CAD build for the part. Positions are in the model's coordinates, mm. Give positions to 0.01 mm unless a question says otherwise; leave off trailing zeros. Loops run counter-clockwise (first coordinate to the right, second up) from the corner with the lowest first, then second, coordinate; pieces in that order, holes last. Notation, with made-up numbers: M -21.75,38 L 3.25,38 A16 cw 3.25,54 Z; hole C 59.5,36.5 d7. An arc over 180 degrees is marked long. Answer as CSV lines item,"result".
```python
from build123d import *

# Parameters (mm, degrees)
F0_R     = 1.7
F1_DEPTH = 5


with BuildPart() as f1:
    # F0 (on Top) → F1 (new body)
    with BuildSketch(Plane.XY):
        with Locations((-11.34986, 17.466265)):
            Circle(F0_R)
        Polygon((-2.84986, 22.466265), (-21.74986, 22.466265), (-21.74986, 12.466265), (-2.84986, 12.466265), (-2.84986, 17.466265), align=None)
        with Locations((-11.34986, 17.466265)):
            Circle(F0_R, mode=Mode.SUBTRACT)
        with BuildLine():
            ThreePointArc((7.35014, 17.466265), (5.65014, 19.166265), (3.95014, 17.466265))
            ThreePointArc((3.95014, 17.466265), (5.65014, 15.766265), (7.35014, 17.466265))
        make_face()
        Polygon((16.05014, 22.466265), (-2.84986, 22.466265), (-2.84986, 17.466265), (-2.84986, 12.466265), (16.05014, 12.466265), align=None)
        with BuildLine():
            ThreePointArc((7.35014, 17.466265), (5.65014, 15.766265), (3.95014, 17.466265))
            ThreePointArc((3.95014, 17.466265), (5.65014, 19.166265), (7.35014, 17.466265))
        make_face(mode=Mode.SUBTRACT)
    extrude(amount=F1_DEPTH)


solid = f1.part
```
Q1. Cut at B-B (x = -11). Write the cut outline in (y, z).
Solution:
outline,"M 12.47,0 L 15.8,0 L 15.8,5 L 12.47,5 Z; M 19.13,0 L 22.47,0 L 22.47,5 L 19.13,5 Z"
Q2. Wall check: line 1 (X direction, y = 18.25, z = 2.85); line 2 (X direction, y = 17, z = 4.3); line 3 (Y direction, x = -10, z = 3.75). Give the ranges that are in metal, low to high. Write a range as [from, to].
Solution:
line 1,"x = [-21.75, -12.86], [-9.84, 4.14], [7.16, 16.05]"
line 2,"x = [-21.75, -12.98], [-9.72, 4.02], [7.28, 16.05]"
line 3,"y = [12.47, 16.43], [18.5, 22.47]"
Q3. Mould opens along Y. For faces 1 (the flat face through (-3, 12.466, 2)), 2 (the cylindrical face through (-10.44, 18.9, 2.46)), 3 (the flat face through (-3, 18, 5)) say: released by +Y, released by -Y, zero draft, split by the parting line, or undercut.
Solution:
face 1,"released by -Y"
face 2,"undercut"
face 3,"zero draft"
Q4. Pin check, flat tips, straight feed: P1, Ø2, axis at x = -11.35, y = 17.47, coming from the +Z side; P2, Ø5.5, axis at x = 5.65, y = 17.47, coming from the +Z side. Stop position of each tip, or through.
Solution:
P1,"passes through"
P2,"stops at z = 5"
Q5. Cut at C-C (z = 4.1). Write the cut outline in (x, y), and give its area (3 significant figures).
Solution:
outline,"M -21.75,12.47 L 16.05,12.47 L 16.05,22.47 L -21.75,22.47 Z; hole C -11.35,17.47 d3.4; hole C 5.65,17.47 d3.4"
area,"360 mm²"
Q6. Cut at A-A (y = 18.75). Write the cut outline in (x, z), and give its area (3 significant figures).
Solution:
outline,"M -21.75,0 L -12.46,0 L -12.46,5 L -21.75,5 Z; M -10.24,0 L 4.54,0 L 4.54,5 L -10.24,5 Z; M 6.76,0 L 16.05,0 L 16.05,5 L 6.76,5 Z"
area,"167 mm²"
Q7. Cut at D-D (y = 16.75). Write the cut outline in (x, z).
Solution:
outline,"M -21.75,0 L -12.89,0 L -12.89,5 L -21.75,5 Z; M -9.81,0 L 4.11,0 L 4.11,5 L -9.81,5 Z; M 7.19,0 L 16.05,0 L 16.05,5 L 7.19,5 Z"
